from build123d import *

# Parameters (mm, degrees)
SKETCH1_R                = 75
BOSS_EXTRUDE1_DEPTH      = 150
SKETCH3_R                = 76
BOSS_EXTRUDE3_DEPTH      = 30
SKETCH4_R                = 76
BOSS_EXTRUDE4_DEPTH      = 5
BOSS_EXTRUDE4_TAPER      = 10
SKETCH5_R                = 75.118365096
BOSS_EXTRUDE5_DEPTH      = 50
BOSS_EXTRUDE6_DEPTH      = 20
BOSS_EXTRUDE6_DEPTH_BACK = 20
SKETCH8_W                = 20
SKETCH8_H                = 15
SKETCH9_W                = 20
SKETCH9_H                = 10
BOSS_EXTRUDE7_DEPTH      = 50
SKETCH10_W               = 20
SKETCH10_H               = 10
BOSS_EXTRUDE8_DEPTH      = 65
SKETCH11_W               = 20
SKETCH11_H               = 10
BOSS_EXTRUDE9_DEPTH      = 50
SKETCH12_W               = 20
SKETCH12_H               = 10
BOSS_EXTRUDE10_DEPTH     = 65
SKETCH13_W               = 20
SKETCH13_H               = 10
BOSS_EXTRUDE11_DEPTH     = 20
SKETCH6_R                = 67.5
CUT_EXTRUDE2_DEPTH       = 200


with BuildPart() as part:
    # Sketch1 → Boss-Extrude1 (new body)
    with BuildSketch(Plane(origin=(0, 0, 0), x_dir=(1, 0, 0), z_dir=(0, 1, 0))):
        with Locations(Location((-42.374837203, 0, 0), (0, 0, 270))):
            Circle(SKETCH1_R)
    extrude(amount=BOSS_EXTRUDE1_DEPTH)

    # Sketch3 → Boss-Extrude3 (add)
    with BuildSketch(Plane(origin=(0, 150, 0), x_dir=(1, 0, 0), z_dir=(0, 1, 0))):
        with Locations(Location((-42.374837203, 0, 0), (0, 0, 270))):
            Circle(SKETCH3_R)
    extrude(amount=BOSS_EXTRUDE3_DEPTH)

    # Sketch4 → Boss-Extrude4 (add)
    with BuildSketch(Plane(origin=(0, 180, 0), x_dir=(1, 0, 0), z_dir=(0, 1, 0))):
        with Locations(Location((-42.374837203, 0, 0), (0, 0, 270))):
            Circle(SKETCH4_R)
    extrude(amount=BOSS_EXTRUDE4_DEPTH, taper=BOSS_EXTRUDE4_TAPER)

    # Sketch5 → Boss-Extrude5 (add)
    with BuildSketch(Plane(origin=(0, 185, 0), x_dir=(1, 0, 0), z_dir=(0, 1, 0))):
        with Locations(Location((-42.374837203, 0, 0), (0, 0, 270))):
            Circle(SKETCH5_R)
    extrude(amount=BOSS_EXTRUDE5_DEPTH)

    # Sketch8 → Boss-Extrude6 (add, two sides: drawn at the far end of the back side and taken through both)
    with BuildSketch(Plane.XY.offset(-80).offset(-BOSS_EXTRUDE6_DEPTH_BACK)):
        with Locations((-4.874837203, 112.5)):
            Rectangle(SKETCH8_W, SKETCH8_H)
        with Locations((-79.874837203, 112.5)):
            Rectangle(SKETCH8_W, SKETCH8_H)
    extrude(amount=BOSS_EXTRUDE6_DEPTH + BOSS_EXTRUDE6_DEPTH_BACK)

    # Sketch9 → Boss-Extrude7 (add)
    with BuildSketch(Plane(origin=(0, 120, 0), x_dir=(1, 0, 0), z_dir=(0, 1, 0))):
        with Locations((-4.874837203, 95)):
            Rectangle(SKETCH9_W, SKETCH9_H)
    extrude(amount=BOSS_EXTRUDE7_DEPTH)

    # Sketch10 → Boss-Extrude8 (add)
    with BuildSketch(Plane(origin=(0, 0, -100), x_dir=(-1, 0, 0), z_dir=(0, 0, -1))):
        with Locations((4.874837203, 165)):
            Rectangle(SKETCH10_W, SKETCH10_H)
    extrude(amount=BOSS_EXTRUDE8_DEPTH)

    # Sketch11 → Boss-Extrude9 (add)
    with BuildSketch(Plane(origin=(0, 120, 0), x_dir=(1, 0, 0), z_dir=(0, 1, 0))):
        with Locations((-79.874837203, 95)):
            Rectangle(SKETCH11_W, SKETCH11_H)
    extrude(amount=BOSS_EXTRUDE9_DEPTH)

    # Sketch12 → Boss-Extrude10 (add)
    with BuildSketch(Plane(origin=(0, 0, -100), x_dir=(-1, 0, 0), z_dir=(0, 0, -1))):
        with Locations((79.874837203, 165)):
            Rectangle(SKETCH12_W, SKETCH12_H)
    extrude(amount=BOSS_EXTRUDE10_DEPTH)

    # Sketch13 → Boss-Extrude11 (add)
    with BuildSketch(Plane.XZ.offset(-160)):
        with Locations((-4.874837203, -160)):
            Rectangle(SKETCH13_W, SKETCH13_H)
        with Locations((-79.874837203, -160)):
            Rectangle(SKETCH13_W, SKETCH13_H)
    extrude(amount=BOSS_EXTRUDE11_DEPTH)

    # Sketch6 → Cut-Extrude2 (cut)
    with BuildSketch(Plane(origin=(0, 235, 0), x_dir=(1, 0, 0), z_dir=(0, 1, 0))):
        with Locations(Location((-42.374837203, 0, 0), (0, 0, 270))):
            Circle(SKETCH6_R)
    extrude(amount=-CUT_EXTRUDE2_DEPTH, mode=Mode.SUBTRACT)


solid = part.part
Geometry: final body of the model. Coordinates: model frame, mm. A direction names the side the tool comes from. Coordinates: 2 decimals unless noted, no trailing zeros. Order: outer loops, then holes, each group sorted by start corner. A loop starts at its lowest first (then second) coordinate and runs counter-clockwise, first axis right, second up.
1) Section A-A (z = 0). Return loops of the section in (x, y), then the cut area to 3 significant figures.
Result sheet:
outline: (-118.37, 150) - (-117.37, 150) - (-117.37, 0) - (32.63, 0) - (32.63, 150) - (33.63, 150) - (33.63, 180) - (32.74, 185) - (32.74, 235) - (25.13, 235) - (25.13, 35) - (-109.87, 35) - (-109.87, 235) - (-117.49, 235) - (-117.49, 185) - (-118.37, 180) - close
area: 8,330 mm2
2) Section B-B (y = 49). Return loops of the section in (x, z).
Result sheet:
outline: circle Ø150 at (-42.37, 0); hole circle Ø135 at (-42.37, 0)
3) Set-up query: faces 1 (the cylindrical face through (-39.072, 209.65, -75.046)), 2 (the flat face through (-5, 105, -80)), 3 (the flat face through (-5, 145, -90)). Return all of +Z, -Z, +X, -X, +Y, -Y with unobstructed straight access to the full face (end or side cutting, diameter ignored); none if empty.
Result sheet:
face 1: +Y
face 2: -Z, +X, -Y
face 3: +X, -X, +Y
4) Draft query along Z for faces 4 (the flat face through (-80, 132, -100)), 5 (the flat face through (-41, 0, -1)), 6 (the flat face through (-5, 150, -155)), 7 (the flat face through (-5, 155, -165)). Return one class per face: released by +Z, released by -Z, zero draft, split by the parting line, or undercut.
Result sheet:
face 4: undercut
face 5: zero draft
face 6: undercut
face 7: released by -Z
5) Ray query, probe 1 along Z at (x, y) = (3, 165.5); probe 2 along X at (y, z) = (133, 0); probe 3 along X at (y, z) = (172.5, 0). Return the intervals inside material, ascending.
Result sheet:
probe 1: z = -165 to -90, -60.97 to -49.97, 49.97 to 60.97
probe 2: x = -117.37 to -109.87, 25.13 to 32.63
probe 3: x = -118.37 to -109.87, 25.13 to 33.63
6) First-contact query: P1, Ø1, axis at y = 76.5, z = 13, coming from the -X side; P2, Ø3, axis at x = -12.5, y = 176.5, coming from the -Z side; P3, Ø22, axis at x = -79.5, z = -139, coming from the +Y side; P4, Ø8, axis at x = -6.5, z = 18, coming from the -Y side. Flat tips, straight axial feed; report the tip coordinate or a pass-through.
Result sheet:
P1: stops at x = -116.33
P2: stops at z = -70.5
P3: stops at y = 170
P4: stops at y = 0
